```python
from build123d import *

# Parameters (mm, degrees)
F0_W      = 59
F0_H      = 88
F1_DEPTH  = 5.3
F2_W      = 57
F2_H      = 86
F3_DEPTH  = 4.8
F4_W      = 12
F4_H      = 4
F5_DEPTH  = 2
F6_W      = 1
F6_H      = 50
F7_DEPTH  = 4
F8_W      = 9
F8_H      = 1
F8_W_2    = 7
F8_H_2    = 1.5
F9_DEPTH  = 4
F10_W     = 16
F10_H     = 3
F11_DEPTH = 1


with BuildPart() as f1:
    # F0 (on Top) → F1 (new body)
    with BuildSketch(Plane.XY):
        Rectangle(F0_W, F0_H)
    extrude(amount=F1_DEPTH)

    # F2 (on face) → F3 (cut)
    with BuildSketch(Plane.XY.offset(5.3)):
        Rectangle(F2_W, F2_H)
    extrude(amount=-F3_DEPTH, mode=Mode.SUBTRACT)

    # F4 (on face) → F5 (cut)
    with BuildSketch(Plane.YZ.offset(-28.5)):
        with Locations((-12, 2.5)):
            Rectangle(F4_W, F4_H)
    extrude(amount=-F5_DEPTH, mode=Mode.SUBTRACT)

    # F6 (on face) → F7 (join)
    with BuildSketch(Plane.XY.offset(0.5)):
        with Locations((-19, 17)):
            Rectangle(F6_W, F6_H)
        with Locations((21, 17)):
            Rectangle(F6_W, F6_H)
    extrude(amount=F7_DEPTH)

    # F8 (on face) → F9 (join)
    with BuildSketch(Plane.XY.offset(0.5)):
        with Locations((-24, 35.330578)):
            Rectangle(F8_W, F8_H)
        with Locations((-24, 5.103508)):
            Rectangle(F8_W, F8_H)
        with Locations((25, 35.330578)):
            Rectangle(F8_W_2, F8_H)
        with Locations((25, 18.469588)):
            Rectangle(F8_W_2, F8_H)
        with Locations((25, -0.5)):
            Rectangle(F8_W_2, F8_H)
        with Locations((-24, 17.75)):
            Rectangle(F8_W, F8_H_2)
    extrude(amount=F9_DEPTH)

    # F10 (on face) → F11 (cut)
    with BuildSketch(Plane.XY.offset(0.5)):
        with Locations((7.3, -20.25)):
            Rectangle(F10_W, F10_H)
    extrude(amount=-F11_DEPTH, mode=Mode.SUBTRACT)


solid = f1.part
```
Geometry: final body of the model. Coordinates: model frame, mm. Coordinates: 2 decimals unless noted, no trailing zeros. Order: outer loops, then holes, each group sorted by start corner. A loop starts at its lowest first (then second) coordinate and runs counter-clockwise, first axis right, second up. Notation, with made-up numbers: (54.5, 64) -> (68.5, 64) arc R8 cw to (68.5, 68) -> close; hole circle Ø2 at (-37.5, 38.25). An arc over 180 degrees is marked (long way). Write each question's results on one line, items separated by ' | '. Start each with the question number.
1) Cut plane C-C, the plane y = -25.5. Output: boundary loops of the cut face in (x, z).
2) First-contact query: pin 1 (6 mm diameter, centred on x = 18.5, y = 5, fed in from +Z); pin 2 (3.5 mm diameter, centred on x = 25.5, y = 10.5, fed in from +Z). Flat tips, straight axial feed; report the tip coordinate or a pass-through.
3) Material intervals for line 1 along Y through (x, z) = (-25, 3.9); line 2 along Y through (x, z) = (22.5, 3.45); line 3 along X through (y, z) = (19, 4.3), sorted ascending.
4) Cut plane D-D, the plane x = -7. Output: boundary loops of the cut face in (y, z), and give its area (3 significant figures).
5) Mould query, pull axis X, two halves, no side actions, for faces 1 (the flat face through (-29.5, -1, 3)), 2 (the flat face through (28.5, -1, 5)), 3 (the flat face through (0, 44, 3)). Classes: released by +X, released by -X, zero draft, split by the parting line, or undercut.
6) Cut plane A-A, the plane x = 0.5. Output: boundary loops of the cut face in (y, z).
7) Cut plane B-B, the plane y = -10.5. Output: boundary loops of the cut face in (x, z), and give its area (3 significant figures).
Checks:
1) outline: (-29.5, 0) -> (29.5, 0) -> (29.5, 5.3) -> (28.5, 5.3) -> (28.5, 0.5) -> (-28.5, 0.5) -> (-28.5, 5.3) -> (-29.5, 5.3) -> close
2) pin 1: z = 4.5 | pin 2: z = 0.5
3) line 1: -44 to -43, 4.6 to 5.6, 17 to 18.5, 34.83 to 35.83, 43 to 44 | line 2: -44 to -43, -1 to 0, 17.97 to 18.97, 34.83 to 35.83, 43 to 44 | line 3: -29.5 to -28.5, -19.5 to -18.5, 20.5 to 21.5, 28.5 to 29.5
4) outline: (-44, 0) -> (44, 0) -> (44, 5.3) -> (43, 5.3) -> (43, 0.5) -> (-43, 0.5) -> (-43, 5.3) -> (-44, 5.3) -> close | area: 53.6 mm^2
5) face 1: released by -X | face 2: undercut | face 3: zero draft
6) outline: (-44, 0) -> (-21.75, 0) -> (-21.75, 0.5) -> (-43, 0.5) -> (-43, 5.3) -> (-44, 5.3) -> close; (-18.75, 0) -> (44, 0) -> (44, 5.3) -> (43, 5.3) -> (43, 0.5) -> (-18.75, 0.5) -> close
7) outline: (-29.5, 0) -> (29.5, 0) -> (29.5, 5.3) -> (28.5, 5.3) -> (28.5, 0.5) -> (-29.5, 0.5) -> close; (-29.5, 4.5) -> (-28.5, 4.5) -> (-28.5, 5.3) -> (-29.5, 5.3) -> close | area: 35.1 mm^2
